Geometry: final body of the model. Coordinates: model frame, mm. A direction names the side the tool comes from. Give positions to 0.01 mm unless a question says otherwise; leave off trailing zeros. Write each loop counter-clockwise with the first axis right and the second up, starting at its lowest first coordinate (ties: lowest second). Pieces come first, ordered by that corner, then holes.
```python
from build123d import *

# Parameters (mm, degrees)
SKETCH_1_R           = 120
EXTRUDE_1_DEPTH      = 15
SKETCH_2_R           = 100
EXTRUDE_2_DEPTH      = 70
SKETCH_3_R           = 80
CUT_EXTRUDE_1_DEPTH  = 70
SKETCH_4_R           = 48.25
CUT_EXTRUDE_2_DEPTH  = 65
EXTRUDE_START        = 30
SKETCH_6_R           = 48.25
EXTRUDE_3_DEPTH      = 12.7
EXTRUDE_4_DEPTH      = 85.7
EXTRUDE_4_DEPTH_BACK = 88.7
SKETCH_8_W           = 57.818005318
SKETCH_8_H           = 12.779998275
FILLET_1_R           = 20
FILLET_2_R           = 20
SKETCH_10_W          = 23.933516112
SKETCH_10_H          = 20
CUT_EXTRUDE_3_DEPTH  = 25
SKETCH_11_R          = 65.278053168
CUT_EXTRUDE_4_DEPTH  = 19
SKETCH_12_W          = 20
SKETCH_12_H          = 14.412930018
CUT_EXTRUDE_5_DEPTH  = 165
SKETCH_13_R          = 1.75
CUT_EXTRUDE_6_DEPTH  = 25


with BuildPart() as part:
    # Sketch 1 → Extrude 1 (new body)
    with BuildSketch(Plane(origin=(0, 0, 0), x_dir=(1, 0, 0), z_dir=(0, 1, 0))):
        with Locations(Location((0, 0, 0), (0, 0, 270))):
            Circle(SKETCH_1_R)
    extrude(amount=EXTRUDE_1_DEPTH)

    # Sketch 2 → Extrude 2 (add)
    with BuildSketch(Plane(origin=(0, 15, 0), x_dir=(1, 0, 0), z_dir=(0, 1, 0))):
        with Locations(Location((0, 0, 0), (0, 0, 270))):
            Circle(SKETCH_2_R)
    extrude(amount=EXTRUDE_2_DEPTH)

    # Sketch 3 → Cut-Extrude 1 (cut)
    with BuildSketch(Plane.XZ):
        with Locations(Location((0, 0, 0), (0, 0, 270))):
            Circle(SKETCH_3_R)
    extrude(amount=-CUT_EXTRUDE_1_DEPTH, mode=Mode.SUBTRACT)

    # Sketch 4 → Cut-Extrude 2 (cut)
    with BuildSketch(Plane(origin=(0, 85, 0), x_dir=(1, 0, 0), z_dir=(0, 1, 0))):
        with Locations(Location((0, 0, 0), (0, 0, 270))):
            Circle(SKETCH_4_R)
    extrude(amount=-CUT_EXTRUDE_2_DEPTH, mode=Mode.SUBTRACT)



with BuildPart() as body_2:
    # Sketch 6 → Extrude 3 (new body)
    with BuildSketch(Plane(origin=(0, 0, 0), x_dir=(1, 0, 0), z_dir=(0, 1, 0)).offset(EXTRUDE_START)):
        with Locations(Location((0, 0, 0), (0, 0, 270))):
            Circle(SKETCH_6_R)
    extrude(amount=EXTRUDE_3_DEPTH)


with BuildPart() as part_1:
    add(part.part)

    add(body_2.part)  # Extrude 4 merges body 2
    # Sketch 8 → Extrude 4 (add, two sides: drawn at the far end of the back side and taken through both)
    with BuildSketch(Plane.XY.offset(-EXTRUDE_4_DEPTH_BACK)):
        with Locations((0.416556234, 36.310000863)):
            Rectangle(SKETCH_8_W, SKETCH_8_H)
    extrude(amount=EXTRUDE_4_DEPTH + EXTRUDE_4_DEPTH_BACK)

    # Fillet 1
    fillet_1_edges = [part_1.edges().sort_by_distance(p)[0] for p in [
        (0.446745886, 29.920001725, 79.998752603),
    ]]
    fillet(fillet_1_edges, radius=FILLET_1_R)

    # Fillet 2
    fillet_2_edges = [part_1.edges().sort_by_distance(p)[0] for p in [
        (14.924805984, 29.920001725, -78.595484389),
    ]]
    fillet(fillet_2_edges, radius=FILLET_2_R)

    # Sketch 10 → Cut-Extrude 3 (cut)
    with BuildSketch(Plane(origin=(0, 85, 0), x_dir=(1, 0, 0), z_dir=(0, 1, 0))):
        with Locations((-59, 0)):
            Rectangle(SKETCH_10_W, SKETCH_10_H)
    extrude(amount=-CUT_EXTRUDE_3_DEPTH, mode=Mode.SUBTRACT)

    # Sketch 11 → Cut-Extrude 4 (cut)
    with BuildSketch(Plane(origin=(0, 85, 0), x_dir=(1, 0, 0), z_dir=(0, 1, 0))):
        Circle(SKETCH_11_R)
    extrude(amount=-CUT_EXTRUDE_4_DEPTH, mode=Mode.SUBTRACT)

    # Sketch 12 → Cut-Extrude 5 (cut)
    with BuildSketch(Plane(origin=(29.325558893, 0, 0), x_dir=(0, 0, -1), z_dir=(1, 0, 0))):
        with Locations((0, 62.793534991)):
            Rectangle(SKETCH_12_W, SKETCH_12_H)
    extrude(amount=-CUT_EXTRUDE_5_DEPTH, mode=Mode.SUBTRACT)

    # Sketch 13 → Cut-Extrude 6 (cut)
    with BuildSketch(Plane.XZ.offset(-29.920001725)):
        with Locations(Location((-8.532886067, 41.634599258, 0), (0, 0, 270))):
            Circle(SKETCH_13_R)
        with Locations(Location((23.406445866, 35.473769068, 0), (0, 0, 270))):
            Circle(SKETCH_13_R)
        with Locations(Location((41.634599258, 8.532886067, 0), (0, 0, 90))):
            Circle(SKETCH_13_R)
        with Locations(Location((35.473769068, -23.406445866, 0), (0, 0, 90))):
            Circle(SKETCH_13_R)
        with Locations(Location((8.532886067, -41.634599258, 0), (0, 0, 270))):
            Circle(SKETCH_13_R)
        with Locations(Location((-23.406445866, -35.473769068, 0), (0, 0, 270))):
            Circle(SKETCH_13_R)
        with Locations(Location((-41.634599258, -8.532886067, 0), (0, 0, 90))):
            Circle(SKETCH_13_R)
        with Locations(Location((-35.473769068, 23.406445866, 0), (0, 0, 90))):
            Circle(SKETCH_13_R)
    extrude(amount=-CUT_EXTRUDE_6_DEPTH, mode=Mode.SUBTRACT)


solid = part_1.part
```
Item 1: Pin query (flat end, axial travel): pin 1 Ø11.5 at (x, y) = (-89, 62.5) entering from -Z; pin 2 Ø16 at (x, z) = (-36, 10) entering from -Y; pin 3 Ø10 at (y, z) = (21, 23.5) entering from +X. Return the tip coordinate at first contact, or that it passes through.
Found:
pin 1: stops at z = -55.4
pin 2: stops at y = 29.92
pin 3: stops at x = 98.27
Item 2: Section B-B, the plane x = 0. Return the cut outline in (y, z), plus the area to 3 significant figures.
Found:
outline: (0, -120) - (15, -120) - (15, -100) - (85, -100) - (85, -65.28) - (70, -65.28) - (70, -80) - (42.7, -80) - (42.7, 80) - (70, 80) - (70, 65.28) - (85, 65.28) - (85, 100) - (15, 100) - (15, 120) - (0, 120) - (0, 80) - (9.92, 80) arc R20 cw to (29.92, 60) - (29.92, -60) arc R20 cw to (9.92, -80) - (0, -80) - close
area: 6,660 mm2
Item 3: Section C-C, the plane y = 19. Return the cut outline in (x, z), plus the area to 3 significant figures.
Found:
outline: circle Ø200 at (0, 0); hole (-28.49, -74.75) - (-28.49, -72.42) arc R77.82 ccw to (29.33, -72.08) - (29.33, -74.43) arc R80 ccw to (29.33, 74.43) - (29.33, 72.08) arc R77.82 ccw to (-28.49, 72.42) - (-28.49, 74.75) arc R80 ccw to start
area: 11,600 mm2
Item 4: Section A-A, the plane z = 0. Return the cut outline in (x, y).
Found:
outline: (-120, 0) - (-80, 0) - (-80, 55.59) - (-100, 55.59) - (-100, 15) - (-120, 15) - close; (-100, 70) - (-70.97, 70) - (-70.97, 85) - (-100, 85) - close; (-48.25, 30) - (-28.49, 30) - (-28.49, 29.92) - (29.33, 29.92) - (29.33, 30) - (48.25, 30) - (48.25, 42.7) - (-48.25, 42.7) - close; (65.28, 70) - (80, 70) - (80, 0) - (120, 0) - (120, 15) - (100, 15) - (100, 85) - (65.28, 85) - close
Item 5: Reachability of faces 1 (the face through (4, 70, 66)), 2 (the face through (-68, 78, 10)), 3 (the face through (98, 15, -27)) from +Z, -Z, +X, -X, +Y, -Y: full face, straight path, thin tool, end or side. Return the list, or none.
Found:
face 1: none
face 2: +Y, -Y
face 3: +Y
Item 6: Section D-D, the plane z = 89. Return the cut outline in (x, y), plus the area to 3 significant figures.
Found:
outline: (-80.49, 0) - (80.49, 0) - (80.49, 15) - (45.6, 15) - (45.6, 85) - (-45.6, 85) - (-45.6, 15) - (-80.49, 15) - close
area: 8,800 mm2
Item 7: Pull-direction query (Y, two-part tool) for faces 4 (the face through (65.22, 77.6, 2.73)), 5 (the face through (-89, 63, -10)), 6 (the face through (0, 29.92, -1)); classes: +Y half, -Y half, draft (parallel to the pull), parting line (faces both ways), or undercut.
Found:
face 4: draft
face 5: undercut
face 6: -Y half
Item 8: Line query: L1, parallel to X at y = 80.75, z = 0; L2, parallel to Y at x = 3, z = 101; L3, parallel to Y at x = -75, z = -18. Output: solid intervals per line, ascending.
Found:
L1: x = -100 to -70.97, 65.28 to 100
L2: y = 0 to 15
L3: y = 70 to 85
